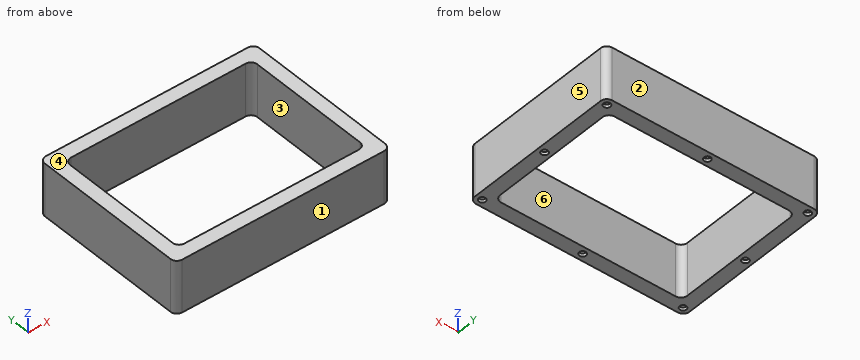
from build123d import *

# Parameters (mm, degrees)
F0_W     = 102
F0_H     = 77
F0_W_2   = 89
F0_H_2   = 64
F1_DEPTH = 25
F2_D     = 3.2
F2_DEPTH = 1.5
F2_TIP   = 0.9613769904
F3_R     = 3


with BuildPart() as f1:
    # F0 (on Top) → F1 (new body)
    with BuildSketch(Plane.XY):
        Rectangle(F0_W, F0_H)
        Rectangle(F0_W_2, F0_H_2, mode=Mode.SUBTRACT)
    extrude(amount=F1_DEPTH)

    # F2
    with Locations(Plane(origin=(0, 0, 0), x_dir=(1, 0, 0), z_dir=(0, 0, -1))):
        with Locations((-47.75, 35.25), (0, 35.25), (47.75, 35.25), (47.75, 0), (47.75, -35.25), (0, -35.25), (-47.75, -35.25), (-47.75, 0)):
            Hole(F2_D / 2, depth=F2_DEPTH)
            with Locations((0, 0, -(F2_DEPTH + F2_TIP / 2))):  # 118° drill point
                Cone(0, F2_D / 2, F2_TIP, mode=Mode.SUBTRACT)

    # F3
    f3_edges = [f1.edges().sort_by_distance(p)[0] for p in [
        (-44.5, -32, 12.5),
        (44.5, -32, 12.5),
        (-44.5, 32, 12.5),
        (44.5, 32, 12.5),
        (-51, -38.5, 12.5),
        (-51, 38.5, 12.5),
        (51, 38.5, 12.5),
        (51, -38.5, 12.5),
    ]]
    fillet(f3_edges, radius=F3_R)


solid = f1.part
Part model, mm, in its own coordinate system. Face numbers are marked on the shaded views. A direction names the side the tool comes from. Round coordinates to 2 decimals unless told otherwise and drop trailing zeros. Loops run counter-clockwise (first coordinate to the right, second up) from the corner with the lowest first, then second, coordinate; pieces in that order, holes last. Notation, with made-up numbers: (74.5, 69) - (111.5, 69) arc R12 cw to (111.5, 87) - close; hole circle Ø3 at (-2, -30.5). An arc over 180 degrees is marked (long way). Answer as a JSON object with one key per item and string values.
Item 1: Band-saw the part on A-A on y = -23. List the corners of the cut face in (x, z), plus the area to 3 significant figures.
Output:
{"outline": "(-51, 0) - (-44.5, 0) - (-44.5, 25) - (-51, 25) - close; (44.5, 0) - (51, 0) - (51, 25) - (44.5, 25) - close", "area": "325 mm2"}
Item 2: Pull direction Y, two halves, no side cores. Call the marked faces 1, 2, 3 and 4: pulls with the +Y half, pulls with the -Y half, needs draft (parallel to the pull), parting line crosses it, or undercut.
Output:
{"face 1": "pulls with the -Y half", "face 2": "pulls with the +Y half", "face 3": "undercut", "face 4": "needs draft"}
Item 3: Band-saw the part on C-C on z = 14.25. List the corners of the cut face in (x, y).
Output:
{"outline": "(-51, -35.5) arc R3 ccw to (-48, -38.5) - (48, -38.5) arc R3 ccw to (51, -35.5) - (51, 35.5) arc R3 ccw to (48, 38.5) - (-48, 38.5) arc R3 ccw to (-51, 35.5) - close; hole (-44.5, -29) arc R3 ccw to (-41.5, -32) - (41.5, -32) arc R3 ccw to (44.5, -29) - (44.5, 29) arc R3 ccw to (41.5, 32) - (-41.5, 32) arc R3 ccw to (-44.5, 29) - close"}
Item 4: Tool access for the marked faces 5 and 6: list every direction of +Z, -Z, +X, -X, +Y, -Y with a clear straight run to the whole face (end or side of a thin tool).
Output:
{"face 5": "+Z, -Z, +X, +Y, -Y", "face 6": "+Z, -Z"}
Item 5: Band-saw the part on B-B on x = 35. List the corners of the cut face in (y, z).
Output:
{"outline": "(-38.5, 0) - (-32, 0) - (-32, 25) - (-38.5, 25) - close; (32, 0) - (38.5, 0) - (38.5, 25) - (32, 25) - close"}
Item 6: Wall check: L1, parallel to Y at x = 0, z = 0.85; L2, parallel to Y at x = 47.75, z = 1.05; L3, parallel to X at y = 35.25, z = 0.95. Give the ranges that are in metal, low to high.
Output:
{"L1": "-38.5 to -36.85, -33.65 to -32, 32 to 33.65, 36.85 to 38.5", "L2": "-38.5 to -36.85, -33.65 to -1.6, 1.6 to 33.65, 36.85 to 38.5", "L3": "-51 to -49.35, -46.15 to -1.6, 1.6 to 46.15, 49.35 to 51"}
Item 7: Pin check, flat tips, straight feed: pin 1 (3.5 mm diameter, centred on x = -47.75, y = -35.25, fed in from -Z); pin 2 (3 mm diameter, centred on x = 47.75, y = -35.25, fed in from -Z). Stop position of each tip, or through.
Output:
{"pin 1": "z = 0", "pin 2": "z = 1.56"}
